from build123d import *

# Parameters (mm, degrees)
SKETCH1_W                  = 21.2
SKETCH1_H                  = 15.1
BOSS_EXTRUDE1_DEPTH        = 2.1
SKETCH2_W                  = 18.8
SKETCH2_H                  = 13
BOSS_EXTRUDE2_DEPTH        = 11.1
BOSS_EXTRUDE3_DEPTH        = 5
BOSS_EXTRUDE3_DEPTH_BACK   = 5
SKETCH14_W                 = 1.495775322
SKETCH14_H                 = 10
CUT_EXTRUDE1_DEPTH         = 5
SKETCH15_R                 = 1.5
CUT_EXTRUDE2_DEPTH         = 0.25
SKETCH16_W                 = 1
SKETCH16_H                 = 5
BOSS_EXTRUDE4_DEPTH        = 9.2
CUT_EXTRUDE3_DEPTH         = 1
CHAMFER1_SIZE              = 1
LPATTERN1_COUNT            = 2
LPATTERN1_PITCH            = 7
LPATTERN1_COUNT_DIR2       = 2
LPATTERN1_PITCH_DIR2       = 7
CHAMFER1_OF_LPATTERN1_SIZE = 1


with BuildPart() as part:
    # Sketch1 → Boss-Extrude1 (new body)
    with BuildSketch(Plane(origin=(0, 0, 0), x_dir=(1, 0, 0), z_dir=(0, 1, 0))):
        Rectangle(SKETCH1_W, SKETCH1_H)
    extrude(amount=BOSS_EXTRUDE1_DEPTH)

    # Sketch2 → Boss-Extrude2 (add)
    with BuildSketch(Plane.XZ):
        Rectangle(SKETCH2_W, SKETCH2_H)
    extrude(amount=BOSS_EXTRUDE2_DEPTH)

    # Sketch12 → Boss-Extrude3 (add, two sides)
    with BuildSketch(Plane.XY) as boss_extrude3_sk:
        Polygon((-8.285775322, 2.1), (5.558513448, 6.1), (6.714224678, 2.1), align=None)
    extrude(amount=BOSS_EXTRUDE3_DEPTH)
    extrude(boss_extrude3_sk.sketch, amount=-BOSS_EXTRUDE3_DEPTH_BACK)

    # Sketch14 → Cut-Extrude1 (cut)
    with BuildSketch(Plane(origin=(0, 2.1, 0), x_dir=(1, 0, 0), z_dir=(0, 1, 0))):
        with Locations((7.462112339, 0)):
            Rectangle(SKETCH14_W, SKETCH14_H)
    extrude(amount=-CUT_EXTRUDE1_DEPTH, mode=Mode.SUBTRACT)

    # Sketch15 → Cut-Extrude2 (cut)
    with BuildSketch(Plane(origin=(-1.198397572, 4.147740514, 0), x_dir=(0.960704213, 0.277574162, 0), z_dir=(-0.277574162, 0.960704213, 0))):
        with Locations((4.033289675, 0)):
            Circle(SKETCH15_R)
    extrude(amount=-CUT_EXTRUDE2_DEPTH, mode=Mode.SUBTRACT)

    # Sketch16 → Boss-Extrude4 (add)
    with BuildSketch(Plane.XZ.offset(11.1)):
        Rectangle(SKETCH16_W, SKETCH16_H)
    boss_extrude4 = extrude(amount=BOSS_EXTRUDE4_DEPTH)

    # Sketch17 → Cut-Extrude3 (cut)
    with BuildSketch(Plane(origin=(0.5, 0, 0), x_dir=(0, 0, -1), z_dir=(1, 0, 0))):
        with BuildLine():
            Line((-0.639644883, -18.511467052), (-0.639644883, -16.117458369))
            ThreePointArc((-0.639644883, -16.117458369), (0, -15.477813486), (0.639644883, -16.117458369))
            Line((0.639644883, -16.117458369), (0.639644883, -18.511467052))
            ThreePointArc((0.639644883, -18.511467052), (0, -19.151111935), (-0.639644883, -18.511467052))
        make_face()
    cut_extrude3 = extrude(amount=-CUT_EXTRUDE3_DEPTH, mode=Mode.SUBTRACT)

    # Chamfer1
    chamfer1_edges = [part.edges().sort_by_distance(p)[0] for p in [
        (0, -20.3, 2.5),
        (0, -20.3, -2.5),
    ]]
    chamfer(chamfer1_edges, length=CHAMFER1_SIZE)

    # LPattern1: Boss-Extrude4, Cut-Extrude3 2 × 2
    with Locations(*[Vector(1, 0, 0) * (i * LPATTERN1_PITCH) + Vector(-1, 0, 0) * (j * LPATTERN1_PITCH_DIR2) for i in range(LPATTERN1_COUNT) for j in range(LPATTERN1_COUNT_DIR2) if (i, j) != (0, 0)]):
        add(boss_extrude4)
        add(cut_extrude3, mode=Mode.SUBTRACT)

    # Chamfer1 of LPattern1
    chamfer1_of_lpattern1_edges = [part.edges().sort_by_distance(p)[0] for p in [
        (-7, -20.3, 2.5),
        (-7, -20.3, -2.5),
        (7, -20.3, 2.5),
        (7, -20.3, -2.5),
        (0, -20.3, 2.5),
        (0, -20.3, -2.5),
    ]]
    chamfer(chamfer1_of_lpattern1_edges, length=CHAMFER1_OF_LPATTERN1_SIZE)


solid = part.part
Here's how the part is built. I have some questions about the finished solid (model axes, mm). A direction names the side the tool comes from. Round coordinates to 2 decimals unless told otherwise and drop trailing zeros. Order: outer loops, then holes, each group sorted by start corner. A loop starts at its lowest first (then second) coordinate and runs counter-clockwise, first axis right, second up. Notation, with made-up numbers: (-21.75, 71.5) -> (23.25, 71.5) arc R15 ccw to (23.25, 90.5) -> close; hole circle Ø8 at (10.25, -6.75). An arc over 180 degrees is marked (long way). Use CSV: the item, a comma, the result in double quotes.
1. I want a section at C-C on y = 0.75. List the corners of the cut face in (x, z) for me, and give its area (3 significant figures).
Recorded:
outline,"(-10.6, -7.55) -> (10.6, -7.55) -> (10.6, 7.55) -> (-10.6, 7.55) -> close; hole (6.71, -5) -> (8.21, -5) -> (8.21, 5) -> (6.71, 5) -> close"
area,"305 mm2"
2. I want a section at A-A on y = -2.5. List the corners of the cut face in (x, z) for me, and give its area (3 significant figures).
Recorded:
outline,"(-9.4, -6.5) -> (9.4, -6.5) -> (9.4, 6.5) -> (-9.4, 6.5) -> close; hole (6.71, -5) -> (8.21, -5) -> (8.21, 5) -> (6.71, 5) -> close"
area,"229 mm2"
3. I'm going to push flat-ended pins straight in: P1, Ø5, axis at y = -11.5, z = -3.5, coming from the +X side; P2, Ø0.5, axis at x = -7, y = -17, coming from the -Z side; P3, Ø0.5, axis at x = 0, y = -14.5, coming from the +Z side; P4, Ø6.5, axis at x = 0.5, z = -2, coming from the -Y side. Where does each tip first touch, or does it pass through?
Recorded:
P1,"stops at x = 9.4"
P2,"stops at z = -2.5"
P3,"stops at z = 2.5"
P4,"stops at y = -20.3"
4. I need wall thicknesses on line 1 along X through (y, z) = (-12.5, 1.75); line 2 along Z through (x, y) = (7, -2.25); line 3 along Z through (x, y) = (0.5, -2.5). Which ranges of each line are inside material? Lowest first, please.
Recorded:
line 1,"x = -7.5 to -6.5, -0.5 to 0.5, 6.5 to 7.5"
line 2,"z = -6.5 to -5, 5 to 6.5"
line 3,"z = -6.5 to 6.5"
5. Thinking about a two-plate mould opening in Z: for faces 5 (the face through (0, -5, -6.5)), 6 (the face through (-7, -17, -0.64)), 7 (the face through (-0.5, -15, 0)), which applies, pulls with the +Z half, pulls with the -Z half, needs draft (parallel to the pull), parting line crosses it, or undercut?
Recorded:
face 5,"pulls with the -Z half"
face 6,"undercut"
face 7,"needs draft"
6. I want a section at D-D on z = 0. Give the number of separate pieces and of enclosed holes in the cut face, and give its area (3 significant figures).
Recorded:
separate pieces,"4"
enclosed holes,"0"
area,"292 mm2"
7. I want a section at B-B on z = 6. List the corners of the cut face in (x, y) for me, and give its area (3 significant figures).
Recorded:
outline,"(-10.6, 0) -> (-9.4, 0) -> (-9.4, -11.1) -> (9.4, -11.1) -> (9.4, 0) -> (10.6, 0) -> (10.6, 2.1) -> (-10.6, 2.1) -> close"
area,"253 mm2"
8. Which directions (+Z, -Z, +X, -X, +Y, -Y) give clear straight access to the entire face, cutting with the end or side of a thin tool? Please do faces 1 (the face through (0, -15, -2.5)), 2 (the face through (0, -17, 0.64)), 3 (the face through (7, 0, 5)), 4 (the face through (7, -15, 2.5)).
Recorded:
face 1,"-Z, +X, -X, -Y"
face 2,"+X, -X"
face 3,"+Y"
face 4,"+Z, +X, -X, -Y"
